Autodesk Inventor part; units mm, degrees
ref_plane "YZ Plane" through (0, 0, 0) normal (1, 0, 0) x (0, 1, 0)
ref_plane "XZ Plane" through (0, 0, 0) normal (0, 1, 0) x (-1, 0, 0)
ref_plane "XY Plane" through (0, 0, 0) normal (0, 0, 1) x (1, 0, 0)
sketch "Sketch1" plane through (0, 0, 0) normal (0, 0, 1) x (1, 0, 0)
  point P0 (0, 0)
sketch "Sketch2" plane through (0, 0, 0) normal (0, 0, 1) x (1, 0, 0)
  line L0 (0, 0) -> (45, 0)
  line L1 (45, 0) -> (45, -105)
  line L2 (45, -105) -> (0, -105)
  line L3 (0, -105) -> (0, 0)
  circle A0 centre (7, -7) radius 1.5
  circle A1 centre (7, -38) radius 1.5
  circle A2 centre (38, -7) radius 1.5
  circle A3 centre (38, -38) radius 1.5
  circle A4 centre (22.5, -22.5) radius 11.5
  dimension "d0" = 45
  dimension "d1" = 105
  dimension "d2" = 3
  dimension "d3" = 3
  dimension "d4" = 3
  dimension "d5" = 3
  dimension "d6" = 31
  dimension "d10" = 7
  dimension "d11" = 7
  dimension "d12" = 31
  dimension "d13" = 7
  dimension "d14" = 7
  dimension "d15" = 31
  dimension "d16" = 31
  dimension "d17" = 23
  dimension "d18" = 22.5
  dimension "d19" = 22.5
extrude "Extrusion1" add sketch "Sketch2" along normal blind 4
sketch "Sketch3" plane through (0, 0, 4) normal (0, 0, 1) x (1, 0, 0)
  point P0 (0, 0)
sketch "Sketch4" plane through (0, 0, 4) normal (0, 0, 1) x (1, 0, 0)
  line L0 (0, 0) -> (0, -105)
  line L1 (45, -105) -> (45, 0)
  line L2 (0, 0) -> (45, 0)
  line L3 (45, 0) -> (45, -105)
  line L4 (45, -105) -> (0, -105)
  line L5 (0, -105) -> (0, 0)
  line L6 (0, -105) -> (45, -105)
  line L7 (45, -105) -> (45, -101)
  line L8 (45, -101) -> (0, -101)
  line L9 (0, -101) -> (0, -105)
  dimension "d22" = 4
extrude "Extrusion2" add sketch "Sketch4" along normal blind 31 contours L8 L1 L4 L0
sketch "Sketch5" plane through (0, -101, 4) normal (0, 1, 0) x (1, 0, 0)
  line L0 (45, 4) -> (0, 4)
  line L1 (45, 4) -> (45, -31)
  line L2 (0, 4) -> (45, 4)
  line L3 (45, 4) -> (45, -31)
  line L4 (45, -31) -> (0, -31)
  line L5 (0, -31) -> (0, 4)
  circle A0 centre (5, -26) radius 1.5
  circle A1 centre (40, -26) radius 1.5
  circle A2 centre (22.5, -6) radius 1.5
  dimension "d25" = 3
  dimension "d26" = 3
  dimension "d27" = 3
  dimension "d28" = 5
  dimension "d29" = 5
  dimension "d30" = 5
  dimension "d31" = 5
  dimension "d32" = 22.5
  dimension "d33" = 25
extrude "Extrusion3" cut sketch "Sketch5" against normal blind 4 contours A0 | A1 | A2
fillet "Fillet1" radius 3 1 edges at (22.5, -101, 4)
fillet "Fillet2" radius 3 1 edges at (0, 0, 2)
fillet "Fillet3" radius 3 1 edges at (0, -103, 35)
fillet "Fillet4" radius 3 1 edges at (45, -103, 35)
fillet "Fillet5" radius 3 1 edges at (45, 0, 2)
properties part number "Suporte Esquerdo 2"
Design review of the part built by this model. Coordinates are the model's own, in mm. A direction names the side the tool comes from. Round coordinates to 2 decimals unless told otherwise and drop trailing zeros. Order: outer loops, then holes, each group sorted by start corner. A loop starts at its lowest first (then second) coordinate and runs counter-clockwise, first axis right, second up. Notation, with made-up numbers: (67.5, 57.25) - (81.5, 57.25) arc R3 cw to (81.5, 61.25) - close; hole circle Ø6 at (21, -39.75). An arc over 180 degrees is marked (long way). Return JSON: item names as keys, results as strings.
Q1. Consider section B-B on x = 9.5. Write out the cut boundary in (y, z).
Computed values:
{"outline": "(-105, 0) - (0, 0) - (0, 4) - (-98, 4) arc R3 cw to (-101, 7) - (-101, 35) - (-105, 35) - close"}
Q2. Consider section A-A on y = -38. Write out the cut boundary in (x, z), plus the area to 3 significant figures.
Computed values:
{"outline": "(0, 0) - (5.5, 0) - (5.5, 4) - (0, 4) - close; (8.5, 0) - (36.5, 0) - (36.5, 4) - (8.5, 4) - close; (39.5, 0) - (45, 0) - (45, 4) - (39.5, 4) - close", "area": "156 mm2"}
Q3. Consider section D-D on x = 16.5. Write out the cut boundary in (y, z).
Computed values:
{"outline": "(-105, 0) - (-32.31, 0) - (-32.31, 4) - (-98, 4) arc R3 cw to (-101, 7) - (-101, 35) - (-105, 35) - close; (-12.69, 0) - (0, 0) - (0, 4) - (-12.69, 4) - close"}
Q4. Consider section C-C on y = -22.5. Write out the cut boundary in (x, z), plus the area to 3 significant figures.
Computed values:
{"outline": "(0, 0) - (11, 0) - (11, 4) - (0, 4) - close; (34, 0) - (45, 0) - (45, 4) - (34, 4) - close", "area": "88.0 mm2"}
Q5. Wall thickness on L1, parallel to X at y = -102.15, z = 30; L2, parallel to Y at x = 38, z = 3; L3, parallel to Z at x = 40, y = -103: over which ranges is each line inside the solid? List them lowest first. Write a range as [from, to].
Computed values:
{"L1": "x = [0, 3.5], [6.5, 38.5], [41.5, 45]", "L2": "y = [-105, -39.5], [-36.5, -8.5], [-5.5, 0]", "L3": "z = [0, 28.5], [31.5, 35]"}
Q6. Machinability: for faces 5 (the flat face through (23, -101, 21)), 6 (the cylindrical face through (36.8, -6.1, 2)), which of the approach directions +Z, -Z, +X, -X, +Y, -Y give a long, thin tool a straight path to every point of the face, cutting with its end or side? Answer none if there is none.
Computed values:
{"face 5": "+Z, +X, -X, +Y", "face 6": "+Z, -Z"}
Q7. The part is to be moulded in two halves that separate along Z. For faces 1 (the cylindrical face through (21.3, -103, 10.9)), 2 (the cylindrical face through (38.89, -102.97, 28.99)), 3 (the flat face through (22, -48, 4)), 4 (the flat face through (23, -105, 17)), say which applies: pulls with the +Z half, pulls with the -Z half, needs draft (parallel to the pull), parting line crosses it, or undercut.
Computed values:
{"face 1": "undercut", "face 2": "undercut", "face 3": "pulls with the +Z half", "face 4": "needs draft"}
Q8. For pin 1 Ø1.5 at (x, z) = (5, 27) entering from +Y; pin 2 Ø3.5 at (x, y) = (7, -7) entering from +Z, all flat-tipped, find the tip position at first contact; note any pin that passes through.
Computed values:
{"pin 1": "stops at y = -101", "pin 2": "stops at z = 4"}
